Here's how the part is built. I have some questions about the finished solid (model axes, mm). A direction names the side the tool comes from. Coordinates: 2 decimals unless noted, no trailing zeros. Order: outer loops, then holes, each group sorted by start corner. A loop starts at its lowest first (then second) coordinate and runs counter-clockwise, first axis right, second up. Notation, with made-up numbers: (-33.75, 2.25) - (14.25, 2.25) arc R20 ccw to (14.25, 10.25) - close; hole circle Ø7 at (82, 47.25). An arc over 180 degrees is marked (long way). Answer in a Markdown table with one row per item. Add a question column.
Item 1: On a 3-axis mill with a long thin cutter (end or side, diameter ignored), from which of +Z, -Z, +X, -X, +Y, -Y can I reach the whole of each face in a straight line? I mean faces 1 (the cylindrical face through (-8.484, -0.528, 0.056)), 2 (the flat face through (0, -7, -5)), 3 (the flat face through (-7.5, -4.4, -4)). Say none if no direction works.
Item 2: Thinking about a two-plate mould opening in X: for faces 4 (the cylindrical face through (-2.17, -9.76, 4.51)), 5 (the cylindrical face through (8.483, -0.539, 0.056)), 6 (the cylindrical face through (-1.06, 8.434, 0.056)), which applies, +X half, -X half, draft (parallel to the pull), parting line (faces both ways), or undercut?
Item 3: Will these pins go through, and if not, where does the flat tip stop? pin 1 Ø0.6 at (x, z) = (0, 1.5) entering from +Y; pin 2 Ø4 at (x, z) = (7.5, 1) entering from -Y; pin 3 Ø4 at (x, z) = (-4.5, -2.5) entering from +Y.
Item 4: I want a section at A-A (x = 0). Please give me the cut outline in (y, z).
Item 5: If I drill on line 1 along Z through (x, y) = (-5.5, 8); line 2 along X through (y, z) = (-1.75, 2); line 3 along X through (y, z) = (-7.5, 2.75), over which ranges is the centre line in solid material (lowest first)? Write a range as from..to.
```python
from build123d import *

# Parameters (mm, degrees)
BOSS_EXTRUDE1_DEPTH = 5
SKETCH2_R           = 10
BOSS_EXTRUDE2_DEPTH = 1
SKETCH4_R           = 6
BOSS_EXTRUDE3_DEPTH = 5
CUT_EXTRUDE1_REACH  = 22.616
SKETCH5_R           = 2.6


with BuildPart() as part:
    # Sketch1 → Boss-Extrude1 (new, symmetric)
    with BuildSketch(Plane.XY):
        with BuildLine():
            Line((-0.4, 9.191300234), (-0.660980834, 8.474261286))
            ThreePointArc((-0.660980834, 8.474261286), (-1.065332485, 8.432974961), (-1.467248177, 8.372406033))
            Line((-1.467248177, 8.372406033), (-1.898350154, 9.002014591))
            Line((-1.898350154, 9.002014591), (-2.673216683, 8.803062681))
            Line((-2.673216683, 8.803062681), (-2.747677989, 8.043647535))
            ThreePointArc((-2.747677989, 8.043647535), (-3.129058698, 7.90310013), (-3.503284589, 7.744481718))
            Line((-3.503284589, 7.744481718), (-4.077419986, 8.247099263))
            Line((-4.077419986, 8.247099263), (-4.77846533, 7.861696324))
            Line((-4.77846533, 7.861696324), (-4.66172843, 7.107621828))
            ThreePointArc((-4.66172843, 7.107621828), (-4.996174644, 6.876644452), (-5.319196746, 6.629943135))
            Line((-5.319196746, 6.629943135), (-6.000290524, 6.973988359))
            Line((-6.000290524, 6.973988359), (-6.583465426, 6.426350674))
            Line((-6.583465426, 6.426350674), (-6.282865329, 5.724998101))
            ThreePointArc((-6.282865329, 5.724998101), (-6.549362564, 5.418103913), (-6.80088421, 5.098820841))
            Line((-6.80088421, 5.098820841), (-7.546140742, 5.262676117))
            Line((-7.546140742, 5.262676117), (-7.974802178, 4.587213776))
            Line((-7.974802178, 4.587213776), (-7.509226693, 3.982651688))
            ThreePointArc((-7.509226693, 3.982651688), (-7.691029946, 3.619123978), (-7.855247106, 3.247320882))
            Line((-7.855247106, 3.247320882), (-8.617839183, 3.220690579))
            Line((-8.617839183, 3.220690579), (-8.865052779, 2.459845366))
            Line((-8.865052779, 2.459845366), (-8.263755727, 1.990060623))
            ThreePointArc((-8.263755727, 1.990060623), (-8.349441631, 1.592741174), (-8.416035937, 1.191779808))
            Line((-8.416035937, 1.191779808), (-9.148047095, 0.976337208))
            Line((-9.148047095, 0.976337208), (-9.198279511, 0.177915826))
            Line((-9.198279511, 0.177915826), (-8.499042597, -0.127573271))
            ThreePointArc((-8.499042597, -0.127573271), (-8.483227192, -0.533719416), (-8.448014278, -0.938645173))
            Line((-8.448014278, -0.938645173), (-9.103449564, -1.32936302))
            Line((-9.103449564, -1.32936302), (-8.953544512, -2.115192821))
            Line((-8.953544512, -2.115192821), (-8.200303363, -2.237191266))
            ThreePointArc((-8.200303363, -2.237191266), (-8.083980389, -2.626644452), (-7.949172812, -3.010091627))
            Line((-7.949172812, -3.010091627), (-8.486848816, -3.551534481))
            Line((-8.486848816, -3.551534481), (-8.146225383, -4.275396123))
            Line((-8.146225383, -4.275396123), (-7.38630891, -4.206238307))
            ThreePointArc((-7.38630891, -4.206238307), (-7.176787367, -4.554527757), (-6.950855584, -4.892402953))
            Line((-6.950855584, -4.892402953), (-7.336988145, -5.550549969))
            Line((-7.336988145, -5.550549969), (-6.827048953, -6.166960564))
            Line((-6.827048953, -6.166960564), (-6.108205503, -5.910991925))
            ThreePointArc((-6.108205503, -5.910991925), (-5.8186504, -6.196233333), (-5.515790536, -6.467306608))
            Line((-5.515790536, -6.467306608), (-5.726117525, -7.200803989))
            Line((-5.726117525, -7.200803989), (-5.078903929, -7.671032191))
            Line((-5.078903929, -7.671032191), (-4.44630108, -7.244336181))
            ThreePointArc((-4.44630108, -7.244336181), (-4.09490623, -7.44860678), (-3.734148082, -7.635845605))
            Line((-3.734148082, -7.635845605), (-3.755453882, -8.398605012))
            Line((-3.755453882, -8.398605012), (-3.011632693, -8.693104654))
            Line((-3.011632693, -8.693104654), (-2.505019208, -8.122492153))
            ThreePointArc((-2.505019208, -8.122492153), (-2.113864041, -8.23295687), (-1.717875372, -8.324596339))
            Line((-1.717875372, -8.324596339), (-1.54882126, -9.068690793))
            Line((-1.54882126, -9.068690793), (-0.755129499, -9.16895738))
            Line((-0.755129499, -9.16895738), (-0.406337766, -8.49028207))
            ThreePointArc((-0.406337766, -8.49028207), (0, -8.5), (0.406337766, -8.49028207))
            Line((0.406337766, -8.49028207), (0.755129499, -9.16895738))
            Line((0.755129499, -9.16895738), (1.54882126, -9.068690793))
            Line((1.54882126, -9.068690793), (1.717875372, -8.324596339))
            ThreePointArc((1.717875372, -8.324596339), (2.113864041, -8.23295687), (2.505019208, -8.122492153))
            Line((2.505019208, -8.122492153), (3.011632693, -8.693104654))
            Line((3.011632693, -8.693104654), (3.755453882, -8.398605012))
            Line((3.755453882, -8.398605012), (3.734148082, -7.635845605))
            ThreePointArc((3.734148082, -7.635845605), (4.09490623, -7.44860678), (4.44630108, -7.244336181))
            Line((4.44630108, -7.244336181), (5.078903929, -7.671032191))
            Line((5.078903929, -7.671032191), (5.726117525, -7.200803989))
            Line((5.726117525, -7.200803989), (5.515790536, -6.467306608))
            ThreePointArc((5.515790536, -6.467306608), (5.8186504, -6.196233333), (6.108205503, -5.910991925))
            Line((6.108205503, -5.910991925), (6.827048953, -6.166960564))
            Line((6.827048953, -6.166960564), (7.336988145, -5.550549969))
            Line((7.336988145, -5.550549969), (6.950855584, -4.892402953))
            ThreePointArc((6.950855584, -4.892402953), (7.176787367, -4.554527757), (7.38630891, -4.206238307))
            Line((7.38630891, -4.206238307), (8.146225383, -4.275396123))
            Line((8.146225383, -4.275396123), (8.486848816, -3.551534481))
            Line((8.486848816, -3.551534481), (7.949172812, -3.010091627))
            ThreePointArc((7.949172812, -3.010091627), (8.083980389, -2.626644452), (8.200303363, -2.237191266))
            Line((8.200303363, -2.237191266), (8.953544512, -2.115192821))
            Line((8.953544512, -2.115192821), (9.103449564, -1.32936302))
            Line((9.103449564, -1.32936302), (8.448014278, -0.938645173))
            ThreePointArc((8.448014278, -0.938645173), (8.483227192, -0.533719416), (8.499042597, -0.127573271))
            Line((8.499042597, -0.127573271), (9.198279511, 0.177915826))
            Line((9.198279511, 0.177915826), (9.148047095, 0.976337208))
            Line((9.148047095, 0.976337208), (8.416035937, 1.191779808))
            ThreePointArc((8.416035937, 1.191779808), (8.349441631, 1.592741174), (8.263755727, 1.990060623))
            Line((8.263755727, 1.990060623), (8.865052779, 2.459845366))
            Line((8.865052779, 2.459845366), (8.617839183, 3.220690579))
            Line((8.617839183, 3.220690579), (7.855247106, 3.247320882))
            ThreePointArc((7.855247106, 3.247320882), (7.691029946, 3.619123978), (7.509226693, 3.982651688))
            Line((7.509226693, 3.982651688), (7.974802178, 4.587213776))
            Line((7.974802178, 4.587213776), (7.546140742, 5.262676117))
            Line((7.546140742, 5.262676117), (6.80088421, 5.098820841))
            ThreePointArc((6.80088421, 5.098820841), (6.549362564, 5.418103913), (6.282865329, 5.724998101))
            Line((6.282865329, 5.724998101), (6.583465426, 6.426350674))
            Line((6.583465426, 6.426350674), (6.000290524, 6.973988359))
            Line((6.000290524, 6.973988359), (5.319196746, 6.629943135))
            ThreePointArc((5.319196746, 6.629943135), (4.996174644, 6.876644452), (4.66172843, 7.107621828))
            Line((4.66172843, 7.107621828), (4.77846533, 7.861696324))
            Line((4.77846533, 7.861696324), (4.077419986, 8.247099263))
            Line((4.077419986, 8.247099263), (3.503284589, 7.744481718))
            ThreePointArc((3.503284589, 7.744481718), (3.129058698, 7.90310013), (2.747677989, 8.043647535))
            Line((2.747677989, 8.043647535), (2.673216683, 8.803062681))
            Line((2.673216683, 8.803062681), (1.898350154, 9.002014591))
            Line((1.898350154, 9.002014591), (1.467248177, 8.372406033))
            ThreePointArc((1.467248177, 8.372406033), (1.065332485, 8.432974961), (0.660980834, 8.474261286))
            Line((0.660980834, 8.474261286), (0.4, 9.191300234))
            Line((0.4, 9.191300234), (-0.4, 9.191300234))
        make_face()
    extrude(amount=BOSS_EXTRUDE1_DEPTH, both=True)

    # Sketch2 → Boss-Extrude2 (add)
    with BuildSketch(Plane.XY.offset(5)):
        Circle(SKETCH2_R)
    boss_extrude2 = extrude(amount=-BOSS_EXTRUDE2_DEPTH)

    # Mirror1: Boss-Extrude2 across plane
    add(boss_extrude2.mirror(Plane.XY))

    # Sketch4 → Boss-Extrude3 (add)
    with BuildSketch(Plane(origin=(0, 0, -5), x_dir=(-1, 0, 0), z_dir=(0, 0, -1))):
        Circle(SKETCH4_R)
    extrude(amount=BOSS_EXTRUDE3_DEPTH)

    # Sketch5 → Cut-Extrude1 (cut, up to next)
    with BuildSketch(Plane.XY.offset(5), mode=Mode.PRIVATE) as cut_extrude1_sk1:
        Circle(SKETCH5_R)
    cut_extrude1_tool1 = extrude(cut_extrude1_sk1.sketch, amount=-CUT_EXTRUDE1_REACH, mode=Mode.PRIVATE) & part.part
    add(cut_extrude1_tool1.solids().sort_by_distance((0, 0, 5))[0], mode=Mode.SUBTRACT)


solid = part.part
```
Values follow:
| question | item | result |
|---|---|---|
| 1 | face 1 | -X |
| 1 | face 2 | -Z |
| 1 | face 3 | none |
| 2 | face 4 | parting line |
| 2 | face 5 | +X half |
| 2 | face 6 | undercut |
| 3 | pin 1 | stops at y = 9.19 |
| 3 | pin 2 | stops at y = -7.37 |
| 3 | pin 3 | stops at y = 9.48 |
| 4 | outline | (-10, -5) - (-6, -5) - (-6, -10) - (-2.6, -10) - (-2.6, 5) - (-10, 5) - (-10, 4) - (-8.5, 4) - (-8.5, -4) - (-10, -4) - close; (2.6, -10) - (6, -10) - (6, -5) - (10, -5) - (10, -4) - (9.19, -4) - (9.19, 4) - (10, 4) - (10, 5) - (2.6, 5) - close |
| 5 | line 1 | z = -5..-4, 4..5 |
| 5 | line 2 | x = -9.02..-1.92, 1.92..9.02 |
| 5 | line 3 | x = -5.31..-4.83, -4..4, 4.83..5.31 |
